Could you check a few things on this model? Use its own coordinates, in mm. Face numbers are marked on the shaded views. A direction names the side the tool comes from. Coordinates: 2 decimals unless noted, no trailing zeros. Loops run counter-clockwise (first coordinate to the right, second up) from the corner with the lowest first, then second, coordinate; pieces in that order, holes last. Notation, with made-up numbers: M 57.25,70 L 65.25,70 A31 ccw 65.25,102 Z; hole C -36.5,23.5 d2. An arc over 180 degrees is marked long. Write each question's results on one line, items separated by ' | '.
```python
from build123d import *

# Parameters (mm, degrees)
BOSS_EXTRUDE1_DEPTH = 25
SKETCH3_R           = 4
CUT_EXTRUDE2_DEPTH  = 228.266363547
CUT_EXTRUDE3_REACH  = 234.056
SKETCH4_R           = 3.4
BOSS_EXTRUDE2_DEPTH = 50
BOSS_EXTRUDE3_DEPTH = 10


with BuildPart() as part:
    # Sketch1 → Boss-Extrude1 (new, symmetric)
    with BuildSketch(Plane.XY):
        Polygon((0, 0), (0, 200), (10, 200), (10, 10), (115, 10), (115, 0), align=None)
    extrude(amount=BOSS_EXTRUDE1_DEPTH, both=True)

    # Sketch3 → Cut-Extrude2 (cut, through all)
    with BuildSketch(Plane(origin=(10, 0, 0), x_dir=(0, 0, -1), z_dir=(1, 0, 0))):
        with Locations((0, 180)):
            Circle(SKETCH3_R)
        with Locations((0, 130)):
            Circle(SKETCH3_R)
        with Locations((0, 80)):
            Circle(SKETCH3_R)
    extrude(amount=-CUT_EXTRUDE2_DEPTH, mode=Mode.SUBTRACT)

    # Sketch4 → Cut-Extrude3 (cut, up to next)
    with BuildSketch(Plane.XZ, mode=Mode.PRIVATE) as cut_extrude3_sk1:
        with Locations(Location((58, 0, 0), (0, 0, 270))):
            Circle(SKETCH4_R)
    cut_extrude3_tool1 = extrude(cut_extrude3_sk1.sketch, amount=-CUT_EXTRUDE3_REACH, mode=Mode.PRIVATE) & part.part
    add(cut_extrude3_tool1.solids().sort_by_distance((58, 0, 0))[0], mode=Mode.SUBTRACT)

    # Sketch5 → Boss-Extrude2 (add)
    with BuildSketch(Plane(origin=(0, 0, -25), x_dir=(-1, 0, 0), z_dir=(0, 0, -1))):
        Polygon((-45, 10), (-10, 10), (-10, 35), align=None)
    extrude(amount=-BOSS_EXTRUDE2_DEPTH)

    # Sketch6 → Boss-Extrude3 (add)
    with BuildSketch(Plane(origin=(0, 0, -25), x_dir=(-1, 0, 0), z_dir=(0, 0, -1))):
        Polygon((-115, 10), (-10, 10), (-10, 35), (-115, 15), align=None)
    boss_extrude3 = extrude(amount=-BOSS_EXTRUDE3_DEPTH)

    # Mirror2: Boss-Extrude3 across plane
    add(boss_extrude3.mirror(Plane(origin=(0, 0, 0), x_dir=(1, 0, 0), z_dir=(0, 0, -1))))


solid = part.part
```
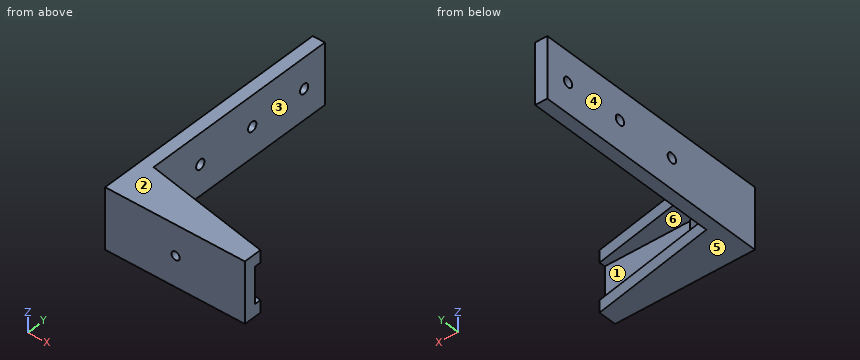
(1) Imagine slicing it at D-D, the plane x = 97.5. List the corners of the cut face in (y, z) for me, and give its area (3 significant figures).
Reported:
outline: M 0,-25 L 18.33,-25 L 18.33,-15 L 10,-15 L 10,15 L 18.33,15 L 18.33,25 L 0,25 Z | area: 667 mm2
(2) If we mould it in two halves opening along Z, with no side actions, what happens to the marked faces 4, 5 and 6? For each: released by +Z, released by -Z, zero draft, split by the parting line, or undercut.
Reported:
face 4: zero draft | face 5: released by -Z | face 6: undercut
(3) Imagine slicing it at C-C, the plane z = -10. List the corners of the cut face in (x, y) for me.
Reported:
outline: M 0,0 L 115,0 L 115,10 L 45,10 L 10,35 L 10,200 L 0,200 Z
(4) Imagine slicing it at B-B, the plane z = 1.5. List the corners of the cut face in (x, y) for me.
Reported:
outline: M 0,0 L 54.95,0 L 54.95,10 L 45,10 L 10,35 L 10,76.29 L 0,76.29 Z; M 0,83.71 L 10,83.71 L 10,126.29 L 0,126.29 Z; M 0,133.71 L 10,133.71 L 10,176.29 L 0,176.29 Z; M 0,183.71 L 10,183.71 L 10,200 L 0,200 Z; M 61.05,0 L 115,0 L 115,10 L 61.05,10 Z
(5) Which directions (+Z, -Z, +X, -X, +Y, -Y) give clear straight access to the entire face, cutting with the end or side of a thin tool? Please do the marked faces 1, 2 and 3.
Reported:
face 1: +X, +Y | face 2: +Z, +X, -X, +Y, -Y | face 3: +Z, -Z, +X, +Y
(6) Please list where these lines run through material, in increasing order: probe 1 along Y at (x, z) = (2.5, 0); probe 2 along X at (y, z) = (110, 18); probe 3 along X at (y, z) = (3, 0). Write a range as from..to.
Reported:
probe 1: y = 0..76, 84..126, 134..176, 184..200 | probe 2: x = 0..10 | probe 3: x = 0..54.6, 61.4..115
(7) Imagine slicing it at A-A, the plane y = 80. List the corners of the cut face in (x, z) for me.
Reported:
outline: M 0,-25 L 10,-25 L 10,-4 L 0,-4 Z; M 0,4 L 10,4 L 10,25 L 0,25 Z
(8) Will these pins go through, and if not, where does the flat tip stop? P1, Ø6.5, axis at y = 130, z = 0, coming from the +X side; P2, Ø10, axis at y = 130.5, z = -8, coming from the -X side; P3, Ø6, axis at x = 65.5, z = 19, coming from the +Y side; P4, Ø15, axis at y = 140, z = 12.5, coming from the +X side.
Reported:
P1: passes through | P2: stops at x = 0 | P3: stops at y = 25 | P4: stops at x = 10
